Read the model definition and answer for the solid it produces. Units are mm, in the model's axes. Face numbers are marked on the shaded views. A direction names the side the tool comes from. Coordinates: 2 decimals unless noted, no trailing zeros. Order: outer loops, then holes, each group sorted by start corner. A loop starts at its lowest first (then second) coordinate and runs counter-clockwise, first axis right, second up. Notation, with made-up numbers: (77.25, 1) - (101.25, 1) arc R11 cw to (101.25, 5) - close; hole circle Ø4 at (27.25, 77.5). An arc over 180 degrees is marked (long way). Use one line per item in the form item = value. Start each with the question number.
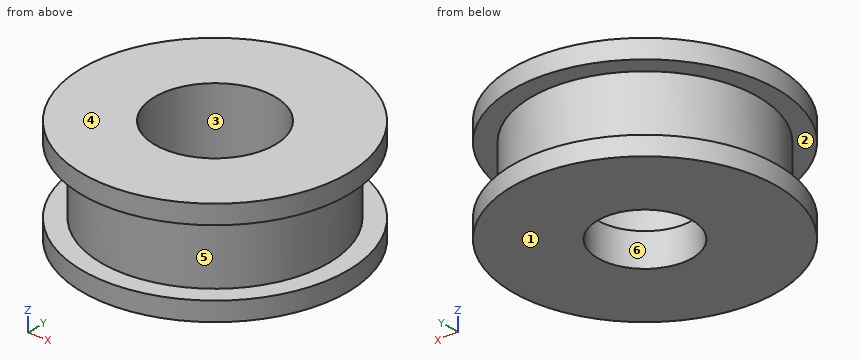
from build123d import *

# Parameters (mm, degrees)
SKETCH1_R            = 14
SKETCH1_R_2          = 12
SKETCH1_R_3          = 2
TOP_FLANGE_DEPTH     = 2
SKETCH1_3_R          = 12
SKETCH1_3_R_2        = 2
CENTER_SPINDLE_DEPTH = 9
BOTTOM_START         = 9
SKETCH1_4_R          = 14
SKETCH1_4_R_2        = 12
SKETCH1_4_R_3        = 2
BOTTOM_FLANGE_DEPTH  = 2
BEARING_START        = -7.5
SKETCH2_R            = 6.35
SKETCH2_R_2          = 5
SKETCH2_R_3          = 2
BEARING_RECESS_DEPTH = 7.5
SKETCH2_3_R          = 5
SKETCH2_3_R_2        = 2
SCREW_OPENING_DEPTH  = 23.649503306


with BuildPart() as part:
    # Sketch1 → Top Flange (new body)
    # profile 1 of 2: a face of its own
    with BuildSketch(Plane.XY):
        Circle(SKETCH1_R)
        Circle(SKETCH1_R_2, mode=Mode.SUBTRACT)
    # profile 2 of 2: a face of its own
    with BuildSketch(Plane.XY):
        Circle(SKETCH1_R_2)
        Circle(SKETCH1_R_3, mode=Mode.SUBTRACT)
    extrude(amount=TOP_FLANGE_DEPTH)

    # Sketch1_3 → Center Spindle (add)
    with BuildSketch(Plane.XY):
        Circle(SKETCH1_3_R)
        Circle(SKETCH1_3_R_2, mode=Mode.SUBTRACT)
    extrude(amount=CENTER_SPINDLE_DEPTH)

    # Sketch1_4 → Bottom Flange (add)
    # profile 1 of 2: a face of its own
    with BuildSketch(Plane.XY.offset(BOTTOM_START)):
        Circle(SKETCH1_4_R)
        Circle(SKETCH1_4_R_2, mode=Mode.SUBTRACT)
    # profile 2 of 2: a face of its own
    with BuildSketch(Plane.XY.offset(BOTTOM_START)):
        Circle(SKETCH1_4_R_2)
        Circle(SKETCH1_4_R_3, mode=Mode.SUBTRACT)
    extrude(amount=BOTTOM_FLANGE_DEPTH)

    # Sketch2 → Bearing Recess (cut)
    # profile 1 of 2: a face of its own
    with BuildSketch(Plane.XY.offset(11).offset(BEARING_START)):
        Circle(SKETCH2_R)
        Circle(SKETCH2_R_2, mode=Mode.SUBTRACT)
    # profile 2 of 2: a face of its own
    with BuildSketch(Plane.XY.offset(11).offset(BEARING_START)):
        Circle(SKETCH2_R_2)
        Circle(SKETCH2_R_3, mode=Mode.SUBTRACT)
    extrude(amount=BEARING_RECESS_DEPTH, mode=Mode.SUBTRACT)

    # Sketch2_3 → Screw Opening (cut, through all)
    with BuildSketch(Plane.XY.offset(11)):
        Circle(SKETCH2_3_R)
        Circle(SKETCH2_3_R_2, mode=Mode.SUBTRACT)
    extrude(amount=-SCREW_OPENING_DEPTH, mode=Mode.SUBTRACT)


solid = part.part
Q1. A cutting plane is placed at D-D (x = -6.75). Give the vertices of the cut face in (y, z), then the cut area to 3 significant figures.
Q2. A cutting plane is placed at C-C (z = 7). Give the vertices of the cut face in (x, y), then the cut area to 3 significant figures.
Q3. Consider probe 1 along Z at (x, y) = (-12.5, 4.75); probe 2 along Y at (x, z) = (0.25, 7.75); probe 3 along Y at (x, z) = (0, 1.95). Determine where each line is inside the solid, lowest interval first.
Q4. Which of the six approach directions +Z, -Z, +X, -X, +Y, -Y give full straight-line access (tool end or side, diameter ignored) to the marked faces 1 and 2?
Q5. A cutting plane is placed at A-A (x = 0). Give the vertices of the cut face in (y, z).
Q6. For a pull along Y with two mould halves and no side action, classify the marked faces 3, 4, 5 and 6 as +Y half, -Y half, draft (parallel to the pull), parting line (faces both ways), or undercut.
Q7. Given P1, Ø6, axis at y = -6.5, z = 9, coming from the -X side; P2, Ø1, axis at x = -5.5, z = 4.5, coming from the -Y side; P3, Ø2, axis at y = 4, z = 7.5, coming from the -X side; P4, Ø4, axis at x = -1, y = -2, coming from the +Z side, each flat-ended and moving along its own axis, determine where each tip first touches the part or whether it passes through.
Result sheet:
q1.outline = (-12.27, 0) - (12.27, 0) - (12.27, 2) - (9.92, 2) - (9.92, 9) - (12.27, 9) - (12.27, 11) - (-12.27, 11) - (-12.27, 9) - (-9.92, 9) - (-9.92, 2) - (-12.27, 2) - close
q1.area = 237 mm^2
q2.outline = circle Ø24 at (0, 0); hole circle Ø12.7 at (0, 0)
q2.area = 326 mm^2
q3.probe_1 = 0 to 2, 9 to 11
q3.probe_2 = -12 to -6.35, 6.35 to 12
q3.probe_3 = -14 to -5, 5 to 14
q4.face_1 = -Z, +X, -X, +Y, -Y
q4.face_2 = none
q5.outline = (-14, 0) - (-5, 0) - (-5, 3.5) - (-6.35, 3.5) - (-6.35, 11) - (-14, 11) - (-14, 9) - (-12, 9) - (-12, 2) - (-14, 2) - close; (5, 0) - (14, 0) - (14, 2) - (12, 2) - (12, 9) - (14, 9) - (14, 11) - (6.35, 11) - (6.35, 3.5) - (5, 3.5) - close
q6.face_3 = undercut
q6.face_4 = draft
q6.face_5 = parting line
q6.face_6 = undercut
q7.P1 = -13.56
q7.P2 = -10.91
q7.P3 = -11.62
q7.P4 = through
